Part model, mm, in its own coordinate system. Face numbers are marked on the shaded views. A direction names the side the tool comes from. Give positions to 0.01 mm unless a question says otherwise; leave off trailing zeros. Write each loop counter-clockwise with the first axis right and the second up, starting at its lowest first coordinate (ties: lowest second). Pieces come first, ordered by that corner, then holes. Notation, with made-up numbers: M 59.5,13.25 L 74.5,13.25 A24 ccw 74.5,43.25 Z; hole C 30,-16 d8. An arc over 180 degrees is marked long. Use CSV: the item, a comma, the result in double quotes. Start each with the question number.
1. Mould opens along X. For the marked faces 1, 2 and 3 say: pulls with the +X half, pulls with the -X half, needs draft (parallel to the pull), parting line crosses it, or undercut.
2. Band-saw the part on C-C, the plane z = 10.5. List the corners of the cut face in (x, y), then the cut area to 3 significant figures.
3. Band-saw the part on D-D, the plane x = 14.5. List the corners of the cut face in (y, z).
4. Band-saw the part on A-A, the plane x = 2.5. List the corners of the cut face in (y, z), then the cut area to 3 significant figures.
5. Drill centre lines: line 1 along X through (y, z) = (2, 3.5); line 2 along X through (y, z) = (1, 11.25); line 3 along Z through (x, y) = (-1, 6). Where is each one in solid material? Low to high. Write a range as from..to.
6. Drop flat-ended pins along their axis: pin 1 Ø5 at (x, z) = (-1.5, 3.5) entering from -Y; pin 2 Ø4 at (x, z) = (-11, 7.5) entering from +Y; pin 3 Ø4 at (x, y) = (-5, 10.5) entering from +Z; pin 4 Ø3 at (x, z) = (-8.5, 10.5) entering from -Y. Give the stop position or say it passes through.
7. Band-saw the part on B-B, the plane y = -5. List the corners of the cut face in (x, z), then the cut area to 3 significant figures.
8. 3-axis set-ups, long thin cutter, end or side, ignore diameter. For the marked faces 4, 5, 6, 7 and 8: which of +Z, -Z, +X, -X, +Y, -Y reach the whole face in a straight line?
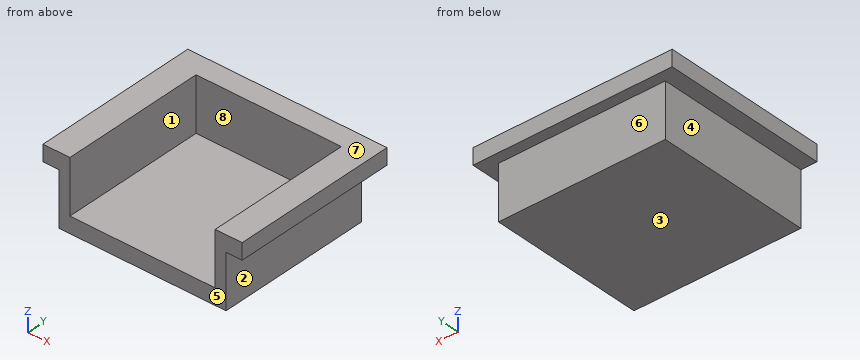
Solid Edge part; units mm, degrees
sketch "Sketch1" plane through (0, 0, 0) normal (0, 0, 1) x (1, 0, 0)
  line L0 (-13.5, -13.5) -> (13.5, -13.5)
  line L1 (13.5, -13.5) -> (13.5, 13.5)
  line L2 (13.5, 13.5) -> (-13.5, 13.5)
  line L3 (-13.5, 13.5) -> (-13.5, -13.5)
extrude "Protrusion1" add sketch "Sketch1" along normal blind 3
sketch "Sketch2" plane through (0, 0, 0) normal (0, 0, -1) x (1, 0, 0)
  line L0 (15.5, 13.5) -> (15.5, -15.5)
  line L1 (15.5, -15.5) -> (-15.5, -15.5)
  line L2 (-15.5, -15.5) -> (-15.5, 13.5)
  line L3 (-15.5, 13.5) -> (-13.5, 13.5)
  line L4 (-13.5, 13.5) -> (-13.5, -13.5)
  line L5 (-13.5, -13.5) -> (13.5, -13.5)
  line L6 (13.5, -13.5) -> (13.5, 13.5)
  line L7 (13.5, 13.5) -> (15.5, 13.5)
extrude "ExtrudedProtrusion_3" add sketch "Sketch2" against normal blind 13
sketch "Sketch3" plane through (0, 1, 13) normal (0, 0, 1) x (1, 0, 0)
  line L0 (13.5, -14.5) -> (26.5, -14.5)
  line L1 (26.5, -14.5) -> (26.5, 19.5)
  line L2 (26.5, 19.5) -> (-28.5, 19.5)
  line L3 (-28.5, 19.5) -> (-28.5, -14.5)
  line L4 (-28.5, -14.5) -> (-13.5, -14.5)
  line L5 (-13.5, -14.5) -> (-13.5, 12.5)
  line L6 (-13.5, 12.5) -> (13.5, 12.5)
  line L7 (13.5, 12.5) -> (13.5, -14.5)
extrude "ExtrudedProtrusion_4" add sketch "Sketch3" against normal blind 3
sketch "Sketch4" plane through (-1, 3.5, 13) normal (0, 0, 1) x (1, 0, 0)
  line L0 (-27.5, -17) -> (-27.5, 17)
  line L1 (-17.5, -17) -> (-27.5, -17)
  line L2 (-17.5, 14) -> (-17.5, -17)
  line L3 (-17.5, 14) -> (19.5, 14)
  line L4 (19.5, -17) -> (19.5, 14)
  line L5 (27.5, -17) -> (19.5, -17)
  line L6 (27.5, 17) -> (27.5, -17)
extrude "Cutout1" cut sketch "Sketch4" against normal up to next material side at (-28.45, 3.5, 13)
Output:
1,face 1,"undercut"
1,face 2,"pulls with the +X half"
1,face 3,"needs draft"
2,outline,"M -18.5,-13.5 L -13.5,-13.5 L -13.5,13.5 L 13.5,13.5 L 13.5,-13.5 L 18.5,-13.5 L 18.5,17.5 L -18.5,17.5 Z"
2,area,"418 mm²"
3,outline,"M -13.5,0 L 15.5,0 L 15.5,10 L 17.5,10 L 17.5,13 L -13.5,13 Z"
4,outline,"M -13.5,0 L 15.5,0 L 15.5,10 L 17.5,10 L 17.5,13 L 13.5,13 L 13.5,3 L -13.5,3 Z"
4,area,"113 mm²"
5,line 1,"x = -15.5..-13.5, 13.5..15.5"
5,line 2,"x = -18.5..-13.5, 13.5..18.5"
5,line 3,"z = 0..3"
6,pin 1,"stops at y = -13.5"
6,pin 2,"stops at y = 15.5"
6,pin 3,"stops at z = 3"
6,pin 4,"stops at y = 13.5"
7,outline,"M -18.5,10 L -15.5,10 L -15.5,0 L 15.5,0 L 15.5,10 L 18.5,10 L 18.5,13 L 13.5,13 L 13.5,3 L -13.5,3 L -13.5,13 L -18.5,13 Z"
7,area,"151 mm²"
8,face 4,"-Z, -X, +Y, -Y"
8,face 5,"+Z, -Z, +X, -X, -Y"
8,face 6,"-Z, +X, -X, +Y"
8,face 7,"+Z, +X, -X, +Y, -Y"
8,face 8,"+Z, -Y"
